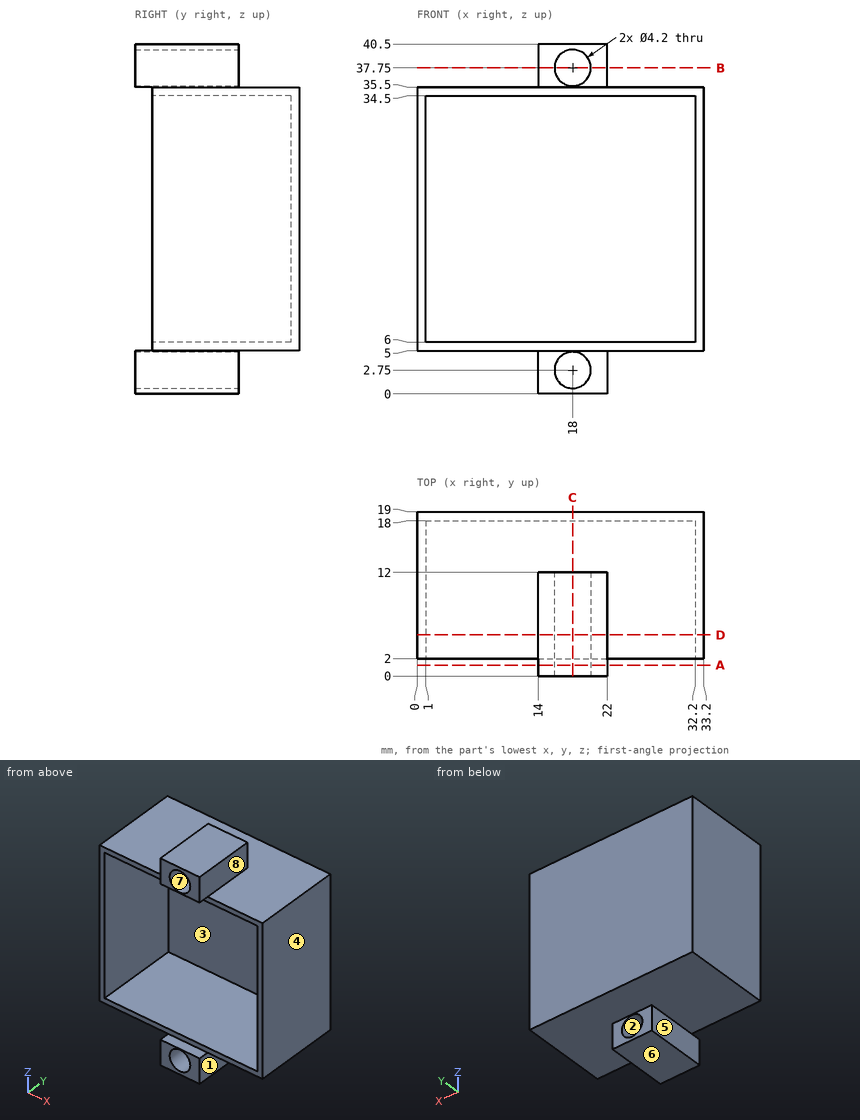
Check sheet for the drawn part. Datum: minimum x, y, z corner. Units: mm. A direction names the side the tool comes from. Coordinates: 2 decimals unless noted, no trailing zeros. Write each loop counter-clockwise with the first axis right and the second up, starting at its lowest first coordinate (ties: lowest second). Pieces come first, ordered by that corner, then holes. Notation, with made-up numbers: (-35.5, 63.5) - (-2.5, 63.5) arc R29 cw to (-2.5, 88.5) - close; hole circle Ø6 at (10.5, 66). An arc over 180 degrees is marked (long way). Answer as a JSON object with one key per item and string values.
(1) Mould release check, pull along X, two halves, no side actions. Record for the marked faces 6, 7 and 8: pulls with the +X half, pulls with the -X half, needs draft (parallel to the pull), parting line crosses it, or undercut.
Report:
{"face 6": "needs draft", "face 7": "undercut", "face 8": "pulls with the +X half"}
(2) Cross-section at D-D on y = 4.75. Record the cut outline in (x, z), plus the area to 3 significant figures.
Report:
{"outline": "(0, 5) - (14, 5) - (14, 0) - (22, 0) - (22, 5) - (33.2, 5) - (33.2, 35.5) - (22, 35.5) - (22, 40.5) - (14, 40.5) - (14, 35.5) - (0, 35.5) - close; hole (1, 6) - (32.2, 6) - (32.2, 34.5) - (1, 34.5) - close; hole circle Ø4.2 at (18, 2.75); hole circle Ø4.2 at (18, 37.75)", "area": "176 mm^2"}
(3) Cross-section at A-A on y = 1.25. Record the cut outline in (x, z).
Report:
{"outline": "(14, 0) - (22, 0) - (22, 5) - (14, 5) - close; (14, 35.5) - (22, 35.5) - (22, 40.5) - (14, 40.5) - close; hole circle Ø4.2 at (18, 2.75); hole circle Ø4.2 at (18, 37.75)"}
(4) Cross-section at C-C on x = 18. Record the cut outline in (y, z), plus the area to 3 significant figures.
Report:
{"outline": "(0, 0) - (12, 0) - (12, 0.65) - (0, 0.65) - close; (0, 4.85) - (12, 4.85) - (12, 5) - (19, 5) - (19, 35.5) - (12, 35.5) - (12, 35.65) - (0, 35.65) - (0, 35.5) - (2, 35.5) - (2, 34.5) - (18, 34.5) - (18, 6) - (2, 6) - (2, 5) - (0, 5) - close; (0, 39.85) - (12, 39.85) - (12, 40.5) - (0, 40.5) - close", "area": "81.7 mm^2"}
(5) Gauge pin test, flat ends, axial feed: pin 1 Ø8 at (x, y) = (10, 14.5) entering from +Z; pin 2 Ø2.5 at (x, z) = (16.5, 39) entering from +Y; pin 3 Ø8.5 at (x, z) = (15, 19) entering from -Y. Record the tip position at first contact, or that the pin passes through.
Report:
{"pin 1": "z = 35.5", "pin 2": "y = 12", "pin 3": "y = 18"}
(6) Cross-section at B-B on z = 37.75. Record the cut outline in (x, y).
Report:
{"outline": "(14, 0) - (15.9, 0) - (15.9, 12) - (14, 12) - close; (20.1, 0) - (22, 0) - (22, 12) - (20.1, 12) - close"}
(7) Thickness scan on line 1 along Z through (x, y) = (18, 8.5); line 2 along Z through (x, y) = (31, 9); line 3 along X through (y, z) = (8.75, 16). Record the ranges inside material, lowest first.
Report:
{"line 1": "0 to 0.65, 4.85 to 6, 34.5 to 35.65, 39.85 to 40.5", "line 2": "5 to 6, 34.5 to 35.5", "line 3": "0 to 1, 32.2 to 33.2"}
(8) Tool access check on the marked faces 1, 2, 3, 4 and 5. Record the directions out of +Z, -Z, +X, -X, +Y, -Y that give a thin tool (end or side, any length) a straight path to the whole face; none if there is none.
Report:
{"face 1": "-Z, +X, +Y, -Y", "face 2": "+Y, -Y", "face 3": "-Y", "face 4": "+Z, -Z, +X, +Y, -Y", "face 5": "-Z, -X, +Y, -Y"}
